Here's how the part is built. I have some questions about the finished solid (model axes, mm). A direction names the side the tool comes from. Round coordinates to 2 decimals unless told otherwise and drop trailing zeros. Loops run counter-clockwise (first coordinate to the right, second up) from the corner with the lowest first, then second, coordinate; pieces in that order, holes last. Notation, with made-up numbers: M -28.75,45 L 26.25,45 A30 cw 26.25,73 Z; hole C 79.25,80 d10. An arc over 180 degrees is marked long. Answer as a JSON object with one key per item and string values.
from build123d import *

# Parameters (mm, degrees)
EXTRUDE003_DEPTH = 110


with BuildPart() as neg_dome:
    # Sketch006 → Revolve002 (revolve)
    with BuildSketch(Plane.XZ):
        with BuildLine():
            add(Edge.make_bspline(
                [(-88.333, 0), (-61.873, 79.23), (0, 75)],
                knots=[0, 0, 0, 1, 1, 1], degree=2))
            Line((0, 75), (0, 0))
            Line((0, 0), (-88.333, 0))
        make_face()
    revolve(axis=Axis((0, 0, 0), (0, 0, 1)))


with BuildPart() as pos_cap:
    # Sketch003 → Extrude003 (new body)
    with BuildSketch(Plane.XZ):
        with BuildLine():
            Line((-47.5, 0), (-47.5, 20.17919))
            ThreePointArc((-27.67919, 40), (-41.694619, 34.194619), (-47.5, 20.17919))
            Line((27.67919, 40), (-27.67919, 40))
            ThreePointArc((47.5, 20.17919), (41.694619, 34.194619), (27.67919, 40))
            Line((47.5, 0), (47.5, 20.17919))
            Line((47.5, 0), (49.5, 0))
            Line((49.5, 0), (49.5, 20.17919))
            ThreePointArc((49.5, 20.17919), (43.108833, 35.608833), (27.67919, 42))
            Line((-27.67919, 42), (27.67919, 42))
            ThreePointArc((-27.67919, 42), (-43.108833, 35.608833), (-49.5, 20.17919))
            Line((-49.5, 0), (-49.5, 20.17919))
            Line((-47.5, 0), (-49.5, 0))
        make_face()
    extrude(amount=EXTRUDE003_DEPTH)

    # Cut002: cut neg_dome
    add(neg_dome.part, mode=Mode.SUBTRACT)


solid = pos_cap.part
Item 1: If we mould it in two halves opening along X, with no side actions, what happens to faces 3 (the face through (0, -86, 42)), 4 (the face through (41.85, -84.61, 34.04)), 5 (the face through (-49.5, -92, 10))? For each: pulls with the +X half, pulls with the -X half, needs draft (parallel to the pull), parting line crosses it, or undercut.
Resolved:
{"face 3": "needs draft", "face 4": "undercut", "face 5": "pulls with the -X half"}
Item 2: Please list where these lines run through material, in increasing order: probe 1 along X at (y, z) = (-75.5, 10); probe 2 along Z at (x, y) = (-25, -82); probe 3 along X at (y, z) = (-77.5, 30). Write a range as from..to.
Resolved:
{"probe 1": "-49.5..-47.5, 47.5..49.5", "probe 2": "40..42", "probe 3": "-47.17..-44.9, 44.9..47.17"}
Item 3: On a 3-axis mill with a long thin cutter (end or side, diameter ignored), from which of +Z, -Z, +X, -X, +Y, -Y can I reach the whole of each face in a straight line? I mean faces 1 (the face through (-41.54, -84.61, 34.35)), 2 (the face through (48, -91, 0)). Say none if no direction works.
Resolved:
{"face 1": "-Z, +Y, -Y", "face 2": "-Z, +X, -X, +Y, -Y"}
Item 4: I want a section at A-A, the plane y = -103.5. Please give me the cut outline in (x, z).
Resolved:
{"outline": "M -49.5,0 L -47.5,0 L -47.5,20.18 A19.82 cw -27.68,40 L 27.68,40 A19.82 cw 47.5,20.18 L 47.5,0 L 49.5,0 L 49.5,20.18 A21.82 ccw 27.68,42 L -27.68,42 A21.82 ccw -49.5,20.18 Z"}
Item 5: I'm going to push flat-ended pins straight in: pin 1 Ø10 at (x, y) = (-38, -87.5) entering from +Z; pin 2 Ø8 at (x, y) = (-16.5, -81.5) entering from -Z; pin 3 Ø1.5 at (x, y) = (-28.5, -104) entering from +Z. Where does each tip first touch, or does it pass through?
Resolved:
{"pin 1": "z = 41.34", "pin 2": "z = 40", "pin 3": "z = 42"}
